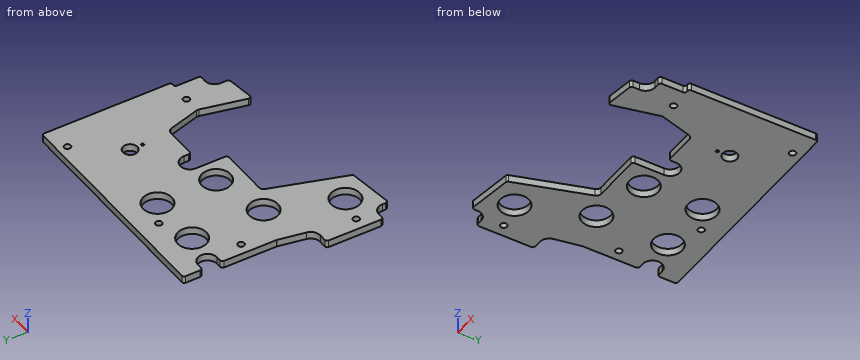
```python
from build123d import *

# Parameters (mm, degrees)
BOSS_EXTRUDE1_DEPTH   = 4.7625
F_6_CLEARANCE_HOLE1_D = 4.3053
SKETCH5_R             = 9.525
SKETCH5_R_2           = 4.7625
CUT_EXTRUDE1_DEPTH    = 5.7625
F_0_CLEARANCE_HOLE1_D = 1.8542


with BuildPart() as part:
    # Sketch1 → Boss-Extrude1 (new body)
    with BuildSketch(Plane.XY):
        with BuildLine():
            Line((-1.58748798, -85.534500226), (-1.587499702, -3.175000338))
            ThreePointArc((-1.587499702, -3.175000338), (-2.052467807, -2.052468316), (-3.174999928, -1.587500451))
            Line((-3.174999928, -1.587500451), (-149.225000608, -1.587521198))
            ThreePointArc((-149.225000608, -1.587521198), (-150.34753241, -2.052489195), (-150.812500382, -3.175021007))
            Line((-150.812500382, -3.175021007), (-150.812501529, -12.700020556))
            ThreePointArc((-150.812501529, -12.700020556), (-150.347533612, -13.822552695), (-149.225001529, -14.287520747))
            Line((-149.225001529, -14.287520747), (-146.049997068, -14.287520747))
            ThreePointArc((-146.049997068, -14.287520747), (-139.699997068, -20.637520747), (-146.049997068, -26.987520747))
            Line((-146.049997068, -26.987520747), (-149.225013631, -26.987520747))
            ThreePointArc((-149.225013631, -26.987520747), (-150.347545646, -27.452488732), (-150.812513631, -28.575020747))
            Line((-150.812513631, -28.575020747), (-150.812513631, -63.3538504))
            ThreePointArc((-150.812513631, -63.3538504), (-150.819200601, -63.499405937), (-150.839205177, -63.643735238))
            Line((-150.839205177, -63.643735238), (-154.094231629, -81.169566712))
            ThreePointArc((-154.094231629, -81.169566712), (-156.277952028, -84.892947063), (-160.337486649, -86.360044427))
            Line((-160.337486649, -86.360044427), (-165.099987777, -86.360045103))
            ThreePointArc((-165.099987777, -86.360045103), (-166.222519646, -86.825013168), (-166.687487552, -87.947545103))
            Line((-166.687487552, -87.947545103), (-166.687487552, -122.545535149))
            ThreePointArc((-166.687487552, -122.545535149), (-166.222519567, -123.668067164), (-165.099987552, -124.133035149))
            Line((-165.099987552, -124.133035149), (-161.924987552, -124.133035149))
            ThreePointArc((-161.924987552, -124.133035149), (-157.434859491, -125.992907088), (-155.574987552, -130.483035149))
            Line((-155.574987552, -130.483035149), (-155.574987552, -132.640440399))
            ThreePointArc((-155.574987552, -132.640440399), (-155.034199033, -133.833986093), (-153.780277221, -134.214359116))
            Line((-153.780277221, -134.214359116), (-125.771097932, -130.526880708))
            ThreePointArc((-125.771097932, -130.526880708), (-124.961326394, -130.171938663), (-124.467007026, -129.438888758))
            Line((-124.467007026, -129.438888758), (-109.180488679, -81.895646464))
            ThreePointArc((-109.180488679, -81.895646464), (-108.028045294, -80.301738907), (-106.157886207, -79.6925))
            Line((-106.157886207, -79.6925), (-74.612491751, -79.6925))
            ThreePointArc((-74.612491751, -79.6925), (-73.489959736, -79.227532015), (-73.024991751, -78.105))
            Line((-73.024991751, -78.105), (-73.024991751, -58.7375))
            ThreePointArc((-73.024991751, -58.7375), (-66.674991751, -52.3875), (-60.324991751, -58.7375))
            Line((-60.324991751, -58.7375), (-60.324991751, -61.9125))
            ThreePointArc((-60.324991751, -61.9125), (-59.860023766, -63.035032015), (-58.737491751, -63.5))
            Line((-58.737491751, -63.5), (-38.786604302, -63.5))
            ThreePointArc((-38.786604302, -63.5), (-36.87752741, -64.138062787), (-35.735764486, -65.795795009))
            Line((-35.735764486, -65.795795009), (-29.83134609, -86.284116742))
            ThreePointArc((-29.83134609, -86.284116742), (-29.708193003, -87.083358908), (-29.790944576, -87.887788459))
            Line((-29.790944576, -87.887788459), (-36.522349245, -116.610151533))
            ThreePointArc((-36.522349245, -116.610151533), (-36.153591729, -118.037818788), (-34.769518371, -118.546303629))
            Line((-34.769518371, -118.546303629), (-17.8902735, -116.324110206))
            ThreePointArc((-17.8902735, -116.324110206), (-16.903937981, -115.796902916), (-16.509983709, -114.750191247))
            Line((-16.509983709, -114.750191247), (-16.509984311, -110.516938696))
            ThreePointArc((-16.509984311, -110.516938696), (-14.655116284, -106.017688645), (-10.160000902, -104.152822935))
            Line((-10.160000902, -104.152822935), (-6.9849852, -104.152822484))
            ThreePointArc((-6.9849852, -104.152822484), (-5.862453251, -103.687854339), (-5.397485425, -102.565322258))
            Line((-5.397485425, -102.565322258), (-5.397487394, -88.709500767))
            ThreePointArc((-5.397487394, -88.709500767), (-4.932519529, -87.586968646), (-3.809987507, -87.122000541))
            Line((-3.809987507, -87.122000541), (-3.17498789, -87.122000474))
            ThreePointArc((-3.17498789, -87.122000474), (-2.052455852, -86.657032363), (-1.58748798, -85.534500226))
        make_face()
    extrude(amount=BOSS_EXTRUDE1_DEPTH)

    # #6 Clearance Hole1 (through all)
    with Locations(Plane.XY.offset(4.7625)):
        with Locations((-103.187497835, -15.240014659), (-18.414998872, -7.937503157), (-143.510001128, -44.450020387), (-158.750001128, -111.125021649), (-18.414987678, -86.741003157)):
            Hole(F_6_CLEARANCE_HOLE1_D / 2)

    # Sketch5 → Cut-Extrude1 (cut, through all)
    with BuildSketch(Plane.XY.offset(4.7625)):
        with Locations((-124.205996572, -24.130021649)):
            Circle(SKETCH5_R)
        with Locations((-87.63, -24.130021649)):
            Circle(SKETCH5_R)
        with Locations((-87.63, -62.992021649)):
            Circle(SKETCH5_R)
        with Locations((-124.205996572, -71.437521424)):
            Circle(SKETCH5_R)
        with Locations((-140.334987552, -115.57)):
            Circle(SKETCH5_R)
        with Locations((-39.36999484, -36.322003157)):
            Circle(SKETCH5_R_2)
    extrude(amount=-CUT_EXTRUDE1_DEPTH, mode=Mode.SUBTRACT)

    # #0 Clearance Hole1 (through all)
    with Locations(Plane.XY.offset(6.35)):
        with Locations((-39.36999484, -44.577003157)):
            Hole(F_0_CLEARANCE_HOLE1_D / 2)


solid = part.part
```
Here's how the part is built. I have some questions about the finished solid (model axes, mm). Coordinates: 2 decimals unless noted, no trailing zeros. Loops run counter-clockwise (first coordinate to the right, second up) from the corner with the lowest first, then second, coordinate; pieces in that order, holes last. Notation, with made-up numbers: M 62.25,81 L 92.25,81 A33 cw 92.25,119 Z; hole C 57,-34 d2. An arc over 180 degrees is marked long. One line per item, written item: value.
1. Imagine slicing it at A-A (x = -87.63). List the corners of the cut face in (y, z) for me.
Geometry says:
outline: M -79.69,0 L -72.52,0 L -72.52,4.76 L -79.69,4.76 Z; M -53.47,0 L -33.66,0 L -33.66,4.76 L -53.47,4.76 Z; M -14.61,0 L -1.59,0 L -1.59,4.76 L -14.61,4.76 Z
2. Will these pins go through, and if not, where does the flat tip stop? pin 1 Ø2.5 at (x, z) = (-163.5, 2) entering from -Y; pin 2 Ø1.3 at (y, z) = (-112.5, 2.5) entering from +X; pin 3 Ø2.5 at (x, z) = (-147, 2.5) entering from -Y; pin 4 Ø3.5 at (x, y) = (-18.41, -7.94) entering from -Z.
Geometry says:
pin 1: stops at y = -124.13
pin 2: stops at x = -16.51
pin 3: stops at y = -133.49
pin 4: passes through
3. Imagine slicing it at C-C (y = -19.5). List the corners of the cut face in (x, z) for me, and give its area (3 significant figures).
Geometry says:
outline: M -139.8,0 L -132.53,0 L -132.53,4.76 L -139.8,4.76 Z; M -115.88,0 L -95.95,0 L -95.95,4.76 L -115.88,4.76 Z; M -79.31,0 L -1.59,0 L -1.59,4.76 L -79.31,4.76 Z
area: 500 mm2
4. Imagine slicing it at B-B (y = -97). List the corners of the cut face in (x, z) for me, and give its area (3 significant figures).
Geometry says:
outline: M -166.69,0 L -114.04,0 L -114.04,4.76 L -166.69,4.76 Z; M -31.93,0 L -5.4,0 L -5.4,4.76 L -31.93,4.76 Z
area: 377 mm2
5. Please list where these lines run through material, in increasing order: probe 1 along Y at (x, z) = (-39.5, 2.8); probe 2 along Y at (x, z) = (-87.63, 3.35); probe 3 along X at (y, z) = (-19, 3.65).
Geometry says:
probe 1: y = -63.5 to -45.49, -43.66 to -41.08, -31.56 to -1.59
probe 2: y = -79.69 to -72.52, -53.47 to -33.66, -14.61 to -1.59
probe 3: x = -139.91 to -132.23, -116.18 to -95.66, -79.6 to -1.59
6. Imagine slicing it at D-D (z = 1). State how many separate pieces and enclosed holes the cut face has, and give its area (3 significant figures).
Geometry says:
separate pieces: 1
enclosed holes: 12
area: 12,600 mm2
